Verification items for the finished model (mm, model axes). A direction names the side the tool comes from. Round coordinates to 2 decimals unless told otherwise and drop trailing zeros. Write each loop counter-clockwise with the first axis right and the second up, starting at its lowest first coordinate (ties: lowest second). Pieces come first, ordered by that corner, then holes. Notation, with made-up numbers: (58.25, 42) - (110.25, 42) arc R28 cw to (110.25, 66) - close; hole circle Ø3 at (10.25, 16.25). An arc over 180 degrees is marked (long way). Answer as a JSON object with one key per item and string values.
```python
from build123d import *

# Parameters (mm, degrees)
CROQUIS2_R              = 2
SALIENTE_EXTRUIR1_DEPTH = 12
SKETCH1_R               = 2
CUT_EXTRUDE1_DEPTH      = 97.1849006


with BuildPart() as part:
    # Croquis2 → Saliente-Extruir1 (new body)
    with BuildSketch(Plane(origin=(0, 0, 0), x_dir=(1, 0, 0), z_dir=(0, 1, 0))):
        with BuildLine():
            Line((-6.5, 70), (-6.5, 0))
            ThreePointArc((-6.5, 0), (0, -6.5), (6.5, 0))
            Line((6.5, 0), (6.5, 24))
            ThreePointArc((6.5, 24), (9.428932188, 31.071067812), (16.5, 34))
            Line((16.5, 34), (19.5, 34))
            Line((19.5, 34), (21.621320344, 36.121320344))
            Line((21.621320344, 36.121320344), (19.621320344, 38.121320344))
            Line((19.621320344, 38.121320344), (21.621320344, 40.121320344))
            Line((21.621320344, 40.121320344), (19.621320344, 42.121320344))
            Line((19.621320344, 42.121320344), (21.621320344, 44.121320344))
            ThreePointArc((21.621320344, 44.121320344), (8.897927721, 59.859277281), (13.535653981, 79.558503244))
            Line((13.535653981, 79.558503244), (11.21874212, 81.180822395))
            Line((11.21874212, 81.180822395), (12.841061271, 83.497734256))
            Line((12.841061271, 83.497734256), (10.524149409, 85.120053407))
            Line((10.524149409, 85.120053407), (12.14646856, 87.436965268))
            Line((12.14646856, 87.436965268), (9.829556699, 89.059284419))
            Line((9.829556699, 89.059284419), (11.451875849, 91.37619628))
            Line((11.451875849, 91.37619628), (11.174038765, 92.951888685))
            Line((11.174038765, 92.951888685), (6.25, 92.083647797))
            Line((6.25, 92.083647797), (-6.5, 70))
        make_face()
        with Locations(Location((0, 0, 0), (0, 0, 270))):
            Circle(CROQUIS2_R, mode=Mode.SUBTRACT)
    extrude(amount=SALIENTE_EXTRUIR1_DEPTH)

    # Sketch1 → Cut-Extrude1 (cut, through all)
    with BuildSketch(Plane(origin=(0, 12, 0), x_dir=(1, 0, 0), z_dir=(0, 1, 0))):
        with Locations(Location((0, 40, 0), (0, 0, 270))):
            Circle(SKETCH1_R)
    extrude(amount=-CUT_EXTRUDE1_DEPTH, mode=Mode.SUBTRACT)


solid = part.part
```
Q1. Set-up check for faces 4 (the flat face through (18, 6, -34)), 5 (the flat face through (11.699, 5.916, -84.298)), 6 (the flat face through (4, 0, -44)): record each of +Z, -Z, +X, -X, +Y, -Y from which the full face is reachable in a straight line by a thin tool's end or side.
Geometry check:
{"face 4": "+Z, +X, +Y, -Y", "face 5": "+X, +Y, -Y", "face 6": "+Z, -Z, +X, -X, -Y"}
Q2. Gauge pin test, flat ends, axial feed: P1, Ø4, axis at y = 9, z = -48, coming from the +X side; P2, Ø6, axis at y = 3.5, z = -10, coming from the +X side; P3, Ø6, axis at x = 16.5, y = 6, coming from the +Z side. Record the tip position at first contact, or that the pin passes through.
Geometry check:
{"P1": "stops at x = 18.32", "P2": "stops at x = 6.5", "P3": "stops at z = -33.54"}
Q3. Section check A-A, the plane y = 8. Record the cut outline in (x, z), then the cut area to 3 significant figures.
Geometry check:
{"outline": "(-6.5, -70) - (6.25, -92.08) - (11.17, -92.95) - (11.45, -91.38) - (9.83, -89.06) - (12.15, -87.44) - (10.52, -85.12) - (12.84, -83.5) - (11.22, -81.18) - (13.54, -79.56) arc R23 cw to (21.62, -44.12) - (19.62, -42.12) - (21.62, -40.12) - (19.62, -38.12) - (21.62, -36.12) - (19.5, -34) - (16.5, -34) arc R10 cw to (6.5, -24) - (6.5, 0) arc R6.5 ccw to (-6.5, 0) - close; hole circle Ø4 at (0, -40); hole circle Ø4 at (0, 0)", "area": "1,490 mm2"}
Q4. Release check for a two-part mould opening along Z. For faces 1 (the flat face through (20.635, 5.916, -37.107)), 2 (the flat face through (-6.5, 6, -35)), 3 (the cylindrical face through (-0.1, 5.9, 6.5)) record: released by +Z, released by -Z, zero draft, split by the parting line, or undercut.
Geometry check:
{"face 1": "undercut", "face 2": "zero draft", "face 3": "released by +Z"}
Q5. Section check B-B, the plane x = 0. Record the cut outline in (y, z).
Geometry check:
{"outline": "(0, -81.26) - (12, -81.26) - (12, -42) - (0, -42) - close; (0, -38) - (12, -38) - (12, -2) - (0, -2) - close; (0, 2) - (12, 2) - (12, 6.5) - (0, 6.5) - close"}
Q6. Section check C-C, the plane z = -5.5. Record the cut outline in (x, y).
Geometry check:
{"outline": "(-6.5, 0) - (6.5, 0) - (6.5, 12) - (-6.5, 12) - close"}
Q7. Section check D-D, the plane x = 4. Record the cut outline in (y, z).
Geometry check:
{"outline": "(0, -88.19) - (12, -88.19) - (12, 5.12) - (0, 5.12) - close"}
Q8. Material ranges on line 1 along X through (y, z) = (4, -40); line 2 along X through (y, z) = (10.5, -21); line 3 along X through (y, z) = (10, -82), recorded low to high. Write a range as [from, to].
Geometry check:
{"line 1": "x = [-6.5, -2], [2, 21.5]", "line 2": "x = [-6.5, 6.5]", "line 3": "x = [0.43, 11.79]"}
